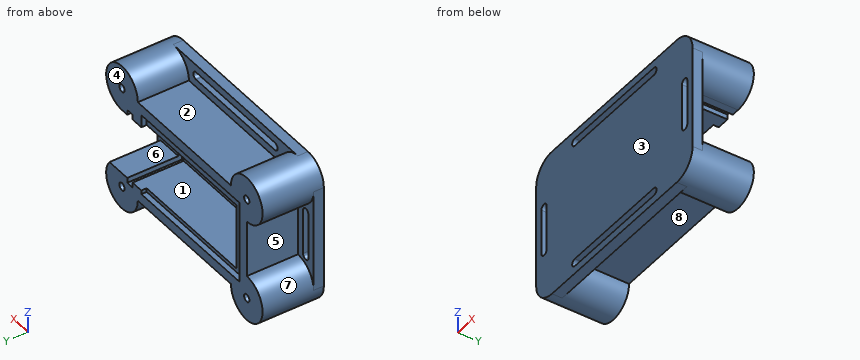
```python
from build123d import *

# Parameters (mm, degrees)
BOSS_EXTRUDE1_DEPTH = 56
SKETCH2_W           = 40.5
SKETCH2_H           = 24.1
BOSS_EXTRUDE2_DEPTH = 4
SKETCH3_W           = 26
SKETCH3_H           = 18
BOSS_EXTRUDE4_DEPTH = 5
BOSS_EXTRUDE5_DEPTH = 11
SKETCH6_W           = 3
SKETCH6_H           = 30
CUT_EXTRUDE1_DEPTH  = 21.6
BOSS_EXTRUDE6_DEPTH = 24.1
BOSS_EXTRUDE7_DEPTH = 4
SKETCH9_R           = 1.5
CUT_EXTRUDE2_DEPTH  = 20


with BuildPart() as part:
    # Sketch1 → Boss-Extrude1 (new body)
    with BuildSketch(Plane(origin=(0, 0, 0), x_dir=(0, 0, -1), z_dir=(1, 0, 0))):
        Polygon((0, 0), (0, -18), (26, -18), (26, 0), (27.5, 0), (27.5, 2.1), (31.5, 2.1), (31.5, -22), (-9, -22), (-9, 2.1), (-5, 2.1), (-5, 0), align=None)
    extrude(amount=-BOSS_EXTRUDE1_DEPTH)

    # Sketch2 → Boss-Extrude2 (add)
    with BuildSketch(Plane.ZY.offset(56)):
        with Locations((-11.25, -9.95)):
            Rectangle(SKETCH2_W, SKETCH2_H)
    extrude(amount=BOSS_EXTRUDE2_DEPTH)

    # Sketch3 → Boss-Extrude4 (add)
    with BuildSketch(Plane(origin=(-56, 0, 0), x_dir=(0, 0, -1), z_dir=(1, 0, 0))):
        with Locations((13, -9)):
            Rectangle(SKETCH3_W, SKETCH3_H)
    extrude(amount=BOSS_EXTRUDE4_DEPTH)

    # Sketch5 → Boss-Extrude5 (add)
    with BuildSketch(Plane(origin=(0, 0, 0), x_dir=(0, 0, -1), z_dir=(1, 0, 0))):
        Polygon((0, 0), (0, 2.1), (-5, 2.1), (-9, 2.1), (-9, -22), (31.5, -22), (31.5, 2.1), (27.5, 2.1), (26, 2.1), (26, 0), (26, -18), (0, -18), align=None)
    extrude(amount=BOSS_EXTRUDE5_DEPTH)

    # Sketch6 → Cut-Extrude1 (cut)
    with BuildSketch(Plane(origin=(0, 2.1, 0), x_dir=(1, 0, 0), z_dir=(0, 1, 0))):
        with Locations((6.5, 13)):
            Rectangle(SKETCH6_W, SKETCH6_H)
    extrude(amount=-CUT_EXTRUDE1_DEPTH, mode=Mode.SUBTRACT)

    # Sketch7 → Boss-Extrude6 (add)
    with BuildSketch(Plane.XZ.offset(22)):
        with BuildLine():
            Line((-60, -22.5), (-60, -31.5))
            Line((-60, -31.5), (-51, -31.5))
            ThreePointArc((-51, -31.5), (-66.363961031, -37.863961031), (-60, -22.5))
        make_face()
        with BuildLine():
            Line((2, -31.5), (11, -31.5))
            Line((11, -31.5), (11, -26))
            Line((11, -26), (18.123903424, -26))
            ThreePointArc((18.123903424, -26), (13.905586789, -40.018072869), (2, -31.5))
        make_face()
        with BuildLine():
            Line((-60, 0), (-60, 9))
            Line((-60, 9), (-51, 9))
            ThreePointArc((-51, 9), (-66.363961031, 15.363961031), (-60, 0))
        make_face()
        with BuildLine():
            Line((2, 9), (11, 9))
            Line((11, 9), (11, 0))
            ThreePointArc((11, 0), (17.363961031, 15.363961031), (2, 9))
        make_face()
    extrude(amount=-BOSS_EXTRUDE6_DEPTH)

    # Sketch8 → Boss-Extrude7 (add)
    with BuildSketch(Plane.XZ.offset(22)):
        with BuildLine():
            Line((11, 18), (-60, 18))
            ThreePointArc((-60, 18), (-53.636038969, 15.363961031), (-51, 9))
            Line((-51, 9), (2, 9))
            ThreePointArc((2, 9), (4.636038969, 15.363961031), (11, 18))
        make_face()
        with BuildLine():
            ThreePointArc((-47, 12), (-48.5, 13.5), (-47, 15))
            Line((-47, 15), (-2, 15))
            ThreePointArc((-2, 15), (-0.5, 13.5), (-2, 12))
            Line((-2, 12), (-47, 12))
        make_face(mode=Mode.SUBTRACT)
        with BuildLine():
            Line((20, -31.5), (20, 9))
            ThreePointArc((20, 9), (17.363961031, 2.636038969), (11, 0))
            Line((11, 0), (11, -26))
            Line((11, -26), (18.123903424, -26))
            ThreePointArc((18.123903424, -26), (19.518072869, -28.594413211), (20, -31.5))
        make_face()
        with BuildLine():
            ThreePointArc((14, -2.25), (15.5, -0.75), (17, -2.25))
            Line((17, -2.25), (17, -20.25))
            ThreePointArc((17, -20.25), (15.5, -21.75), (14, -20.25))
            Line((14, -20.25), (14, -2.25))
        make_face(mode=Mode.SUBTRACT)
        with BuildLine():
            ThreePointArc((-51, -31.5), (-53.636038969, -37.863961031), (-60, -40.5))
            Line((-60, -40.5), (11, -40.5))
            ThreePointArc((11, -40.5), (4.636038969, -37.863961031), (2, -31.5))
            Line((2, -31.5), (-51, -31.5))
        make_face()
        with BuildLine():
            ThreePointArc((-47, -37.5), (-48.5, -36), (-47, -34.5))
            Line((-47, -34.5), (-2, -34.5))
            ThreePointArc((-2, -34.5), (-0.5, -36), (-2, -37.5))
            Line((-2, -37.5), (-47, -37.5))
        make_face(mode=Mode.SUBTRACT)
        with BuildLine():
            ThreePointArc((-60, 0), (-66.363961031, 2.636038969), (-69, 9))
            Line((-69, 9), (-69, -31.5))
            ThreePointArc((-69, -31.5), (-66.363961031, -25.136038969), (-60, -22.5))
            Line((-60, -22.5), (-60, 0))
        make_face()
        with BuildLine():
            ThreePointArc((-63, -20.25), (-64.5, -21.75), (-66, -20.25))
            Line((-66, -20.25), (-66, -2.25))
            ThreePointArc((-66, -2.25), (-64.5, -0.75), (-63, -2.25))
            Line((-63, -2.25), (-63, -20.25))
        make_face(mode=Mode.SUBTRACT)
    extrude(amount=-BOSS_EXTRUDE7_DEPTH)

    # Sketch9 → Cut-Extrude2 (cut)
    with BuildSketch(Plane(origin=(0, 2.1, 0), x_dir=(1, 0, 0), z_dir=(0, 1, 0))):
        with Locations((11, 31.5)):
            Circle(SKETCH9_R)
        with Locations((-60, 31.5)):
            Circle(SKETCH9_R)
        with Locations((-60, -9)):
            Circle(SKETCH9_R)
        with Locations((11, -9)):
            Circle(SKETCH9_R)
    extrude(amount=-CUT_EXTRUDE2_DEPTH, mode=Mode.SUBTRACT)


solid = part.part
```
Work out the finished part from the listing and answer in its coordinate system (mm). Face numbers are marked on the shaded views. A direction names the side the tool comes from. Coordinates: 2 decimals unless noted, no trailing zeros. Write each loop counter-clockwise with the first axis right and the second up, starting at its lowest first coordinate (ties: lowest second). Pieces come first, ordered by that corner, then holes. Notation, with made-up numbers: (72, 14) - (81, 14) arc R17 cw to (81, 45) - close; hole circle Ø6 at (-32, 49.5). An arc over 180 degrees is marked (long way). Answer as a JSON object with one key per item and string values.
Q1. Find section C-C (y = -12.25). Write down the section's boundary in (x, z), plus the area to 3 significant figures.
Results list:
{"outline": "(-60, -22.5) arc R9 ccw (long way) to (-51, -31.5) - (2, -31.5) arc R9 ccw (long way) to (18.12, -26) - (8, -26) - (8, -28) - (5, -28) - (5, -26) - (-51, -26) - (-51, 0) - (5, 0) - (5, 2) - (8, 2) - (8, 0) - (11, 0) arc R9 ccw (long way) to (2, 9) - (-51, 9) arc R9 ccw (long way) to (-60, 0) - close; hole circle Ø3 at (-60, -31.5); hole circle Ø3 at (-60, 9); hole circle Ø3 at (11, -31.5); hole circle Ø3 at (11, 9)", "area": "1,970 mm^2"}
Q2. Find section D-D (x = 15.5). Write down the section's boundary in (y, z), plus the area to 3 significant figures.
Results list:
{"outline": "(-22, -39.29) - (2.1, -39.29) - (2.1, -26) - (-18, -26) - (-18, -21.75) - (-22, -21.75) - close; (-22, -0.75) - (-18, -0.75) - (-18, 1.21) - (2.1, 1.21) - (2.1, 16.79) - (-22, 16.79) - close", "area": "721 mm^2"}
Q3. Find section A-A (z = -4.5). Write down the section's boundary in (x, y).
Results list:
{"outline": "(-69, -22) - (-66, -22) - (-66, -18) - (-69, -18) - close; (-63, -22) - (14, -22) - (14, -18) - (8, -18) - (8, -19.5) - (5, -19.5) - (5, -18) - (-51, -18) - (-51, 0) - (-56, 0) - (-56, 2.1) - (-60, 2.1) - (-60, -18) - (-63, -18) - close; (17, -22) - (20, -22) - (20, -18) - (17, -18) - close"}
Q4. Consider L1, parallel to Z at x = 11, y = -11.25; L2, parallel to Z at x = -38, y = -2.75; L3, parallel to X at y = -7.75, z = -32.5. Determine where each line is inside the solid, lowest interval first. Write a range as from..to.
Results list:
{"L1": "z = -40.5..-33, -30..-26, 0..7.5, 10.5..18", "L2": "z = -31.5..-26, 0..9", "L3": "x = -68.94..-61.12, -58.88..-51.06, 2.06..9.88, 12.12..19.94"}
Q5. Given pin 1 Ø1.5 at (x, y) = (-23.5, -3.5) entering from +Z; pin 2 Ø3 at (x, y) = (14.5, -10.5) entering from +Z; pin 3 Ø2.5 at (x, z) = (7, -11.5) entering from +Y, each flat-ended and moving along its own axis, determine where each tip first touches the part or whether it passes through.
Results list:
{"pin 1": "stops at z = 9", "pin 2": "stops at z = 17.77", "pin 3": "stops at y = -18"}
Q6. Find section B-B (x = -34). Write down the section's boundary in (y, z).
Results list:
{"outline": "(-22, -40.5) - (-18, -40.5) - (-18, -37.5) - (-22, -37.5) - close; (-22, -34.5) - (-18, -34.5) - (-18, -31.5) - (2.1, -31.5) - (2.1, -27.5) - (0, -27.5) - (0, -26) - (-18, -26) - (-18, 0) - (0, 0) - (0, 5) - (2.1, 5) - (2.1, 9) - (-18, 9) - (-18, 12) - (-22, 12) - close; (-22, 15) - (-18, 15) - (-18, 18) - (-22, 18) - close"}
Q7. For a pull along Z with two mould halves and no side action, classify the marked faces 1, 2 and 3 as pulls with the +Z half, pulls with the -Z half, needs draft (parallel to the pull), parting line crosses it, or undercut.
Results list:
{"face 1": "undercut", "face 2": "pulls with the +Z half", "face 3": "needs draft"}
Q8. Which of the six approach directions +Z, -Z, +X, -X, +Y, -Y give full straight-line access (tool end or side, diameter ignored) to the marked faces 4, 5, 6, 7 and 8?
Results list:
{"face 4": "+Z, -Z, +X, -X, +Y", "face 5": "-X, +Y", "face 6": "+X, +Y", "face 7": "+Y", "face 8": "-Z, +Y"}
